Source: CAD feature listing. Evaluate the final solid. Frame: model axes, mm. Face numbers are marked on the shaded views. A direction names the side the tool comes from. Coordinates: 2 decimals unless noted, no trailing zeros. Order: outer loops, then holes, each group sorted by start corner. A loop starts at its lowest first (then second) coordinate and runs counter-clockwise, first axis right, second up. Notation, with made-up numbers: (-4.5, 62) - (54.5, 62) arc R11 ccw to (54.5, 78) - close; hole circle Ø9 at (34.25, 73). An arc over 180 degrees is marked (long way). One line per question, with ' | ' between items. Start each with the question number.
(1) Section D-D (y = -7). Return the cut outline in (x, z) (1 decimal).
(2) Section C-C (z = -6.5). Return the cut outline in (x, y) (1 decimal), then the cut area to 3 significant figures.
(3) Section A-A (x = 11.5). Return the cut outline in (y, z), then the cut area to 3 significant figures.
(4) Line query: line 1 along X through (y, z) = (0, 3); line 2 along X through (y, z) = (0, 5.25); line 3 along Z through (x, y) = (10, 0). Output: solid intervals per line, ascending.
(5) Draft query along Y for the marked faces 1, 2, 3 and 4. Return one class per face: +Y half, -Y half, draft (parallel to the pull), parting line (faces both ways), or undercut.
(6) Contact query for flat-ended pins moving along their axis: P1, Ø6.5, axis at y = 0, z = 0, coming from the +X side; P2, Ø6, axis at x = 11.5, z = 7, coming from the +Y side; P3, Ø1.5, axis at x = 27, z = -1, coming from the +Y side; P4, Ø4, axis at x = 19, y = -1.5, coming from the +Z side. Output: stop coordinate, or through.
(7) Section B-B (y = 0). Count the separate pieces of the cut face and the enclosed holes in it, then the cut area to 3 significant figures.
(8) Access query for the marked faces 5, 6 and 7. Directions: +Z, -Z, +X, -X, +Y, -Y. A direction counts if a zero-diameter tool reaches every point of the face in a straight line with its end or side. Return the directions, or none.
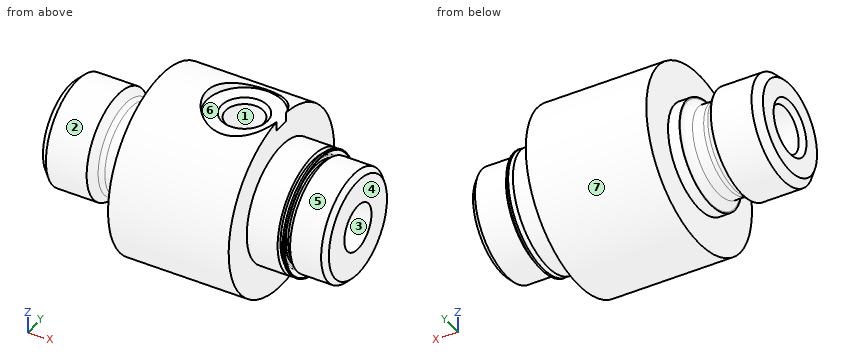
Autodesk Inventor part; units mm, degrees
ref_plane "dp1_XY" through (9.525, 5.5245, 0) normal (0, 0, 1) x (1, 0, 0)
ref_plane "dp1_YZ" through (9.525, 5.5245, 0) normal (1, 0, 0) x (0, 1, 0)
ref_plane "dp1_ZX" through (9.525, 5.5245, 0) normal (0, 1, 0) x (0, 0, 1)
sketch "Sketch_2" plane through (0, 0, 0) normal (0, 0, 1) x (1, 0, 0)
  line L0 (9.525, 0) -> (0, 0)
  line L1 (0, 0) -> (0, 4.8006)
  line L2 (0, 4.8006) -> (0.7557, 5.5563)
  line L3 (0.7557, 5.5563) -> (5.0286, 5.5563)
  line L4 (5.0286, 5.5563) -> (5.7864, 4.8042)
  arc A0 (5.7864, 4.8042) -> (6.35, 4.572) centre (6.35, 5.3721) ccw
  line L5 (6.35, 4.572) -> (7.5184, 4.572)
  arc A1 (7.5184, 4.572) -> (8.3185, 5.3721) centre (7.5184, 5.3721) ccw
  line L6 (8.3185, 5.3721) -> (8.3185, 5.5245)
  line L7 (8.3185, 5.5245) -> (9.525, 5.5245)
  line L8 (9.525, 5.5245) -> (9.525, 0)
  line L9 (9.525, 0) -> (0, 0)
revolve "Revolution1" add sketch "Sketch_2" angle 360 about axis through (9.525, 0, 0) along (1, 0, 0)
thread "Thread1"
sketch "Sketch_3" plane through (0, 0, 0) normal (0, 0, 1) x (1, 0, 0)
  line L0 (30.1752, 0) -> (9.525, 0)
  line L1 (9.525, 0) -> (9.525, 9.3726)
  line L2 (9.525, 9.3726) -> (25.4, 9.3726)
  line L3 (25.4, 9.3726) -> (25.4, 5.1626)
  line L4 (25.4, 5.1626) -> (25.908, 5.1626)
  line L5 (25.908, 5.1626) -> (26.416, 5.6706)
  line L6 (26.416, 5.6706) -> (29.6672, 5.6706)
  line L7 (29.6672, 5.6706) -> (30.1752, 5.1626)
  line L8 (30.1752, 5.1626) -> (30.1752, 0)
  line L9 (30.1752, 0) -> (9.525, 0)
revolve "Revolution2" add sketch "Sketch_3" angle 360 about axis through (30.1752, 0, 0) along (1, 0, 0)
sketch "Sketch3" plane through (0, 0, 0) normal (-1, 0, 0) x (0, 0, 1)
  point P0 (0, 0)
hole "Hole1" at (0, 0, 0) direction (1, 0, 0) diameter 4.8133 depth 30.1752 countersink diameter 5.8293 countersink angle 90
sketch "Sketch_12" plane through (0, 0, 0) normal (0, 1, 0) x (-1, 0, 0)
  line L0 (-18.288, 9.3726) -> (-18.288, -1.016)
  line L1 (-18.288, -1.016) -> (-20.2717, -1.016)
  line L2 (-20.2717, -1.016) -> (-20.2717, 7.9273)
  line L3 (-20.2717, 7.9273) -> (-20.701, 8.3566)
  line L4 (-20.701, 8.3566) -> (-22.2504, 8.3566)
  line L5 (-22.2504, 8.3566) -> (-22.2504, 9.3726)
  line L6 (-22.2504, 9.3726) -> (-18.288, 9.3726)
  line L7 (-18.288, 9.3726) -> (-18.288, -1.016)
revolve "Revolution3" cut sketch "Sketch_12" angle 360 about axis through (18.288, 0, 9.3726) along (0, 0, 1)
thread "Thread2"
sketch "Sketch_14" plane through (0, 0, 0) normal (0, 0, 1) x (1, 0, 0)
  line L0 (25.4, 0) -> (22.1615, 0)
  line L1 (22.1615, 6.1659) -> (25.4, 6.1659)
  line L2 (25.4, 6.1659) -> (25.4, 9.9758)
  line L3 (25.4, 9.9758) -> (22.1615, 9.9758)
  line L4 (22.1615, 9.9758) -> (22.1615, 6.1659)
revolve "Revolution4" cut sketch "Sketch_14" angle 360 about axis through (25.4, 0, 0) along (1, 0, 0)
sketch "Sketch_47" plane through (0, 0, 0) normal (0, 0, 1) x (1, 0, 0)
  line L0 (25.908, 0) -> (25.4, 0)
  line L1 (25.4, 4.9085) -> (25.908, 4.9085)
  line L2 (25.908, 4.9085) -> (25.908, 5.1626)
  line L3 (25.908, 5.1626) -> (25.654, 5.1626)
  line L4 (25.654, 5.1626) -> (25.5116, 5.305)
  arc A0 (25.5116, 5.4846) -> (25.5116, 5.305) centre (25.6014, 5.3948) ccw
  line L5 (25.5116, 5.4846) -> (26.1087, 6.0817)
  line L6 (26.1087, 6.0817) -> (26.1087, 6.1659)
  line L7 (26.1087, 6.1659) -> (25.9055, 6.1659)
  line L8 (25.9055, 6.1659) -> (25.4, 5.6603)
  line L9 (25.4, 5.6603) -> (25.4, 4.9085)
revolve "Revolution5" add sketch "Sketch_47" angle 360 about axis through (25.908, 0, 0) along (1, 0, 0)
ref_plane "dp1_XY" through (9.525, 5.5245, 0) normal (0, 0, 1) x (1, 0, 0)
ref_plane "dp1_YZ" through (9.525, 5.5245, 0) normal (1, 0, 0) x (0, 1, 0)
ref_plane "dp1_ZX" through (9.525, 5.5245, 0) normal (0, 1, 0) x (0, 0, 1)
ref_plane "dp2_XY" through (9.525, -5.5245, 0) normal (0, 0, 1) x (1, 0, 0)
ref_plane "dp2_YZ" through (9.525, -5.5245, 0) normal (1, 0, 0) x (0, 1, 0)
ref_plane "dp2_ZX" through (9.525, -5.5245, 0) normal (0, 1, 0) x (0, 0, 1)
ref_plane "port_XY" through (18.288, 0, 0) normal (0, 0, 1) x (1, 0, 0)
ref_plane "port_YZ" through (18.288, 0, 0) normal (1, 0, 0) x (0, 1, 0)
ref_plane "port_ZX" through (18.288, 0, 0) normal (0, 1, 0) x (0, 0, 1)
ref_plane "rod_guide_XY" through (0, 0, 0) normal (1, 0, 0) x (0, 0, -1)
ref_plane "rod_guide_YZ" through (0, 0, 0) normal (0, 0, -1) x (0, 1, 0)
ref_plane "rod_guide_ZX" through (0, 0, 0) normal (0, 1, 0) x (1, 0, 0)
ref_plane "s1_XY" through (8.3185, 0, 0) normal (0, 0, 1) x (1, 0, 0)
ref_plane "s1_YZ" through (8.3185, 0, 0) normal (1, 0, 0) x (0, 1, 0)
ref_plane "s1_ZX" through (8.3185, 0, 0) normal (0, 1, 0) x (0, 0, 1)
ref_plane "s2_XY" through (9.525, 0, 0) normal (0, 0, 1) x (1, 0, 0)
ref_plane "s2_YZ" through (9.525, 0, 0) normal (1, 0, 0) x (0, 1, 0)
ref_plane "s2_ZX" through (9.525, 0, 0) normal (0, 1, 0) x (0, 0, 1)
ref_plane "t1_XY" through (9.525, 0, 0) normal (1, 0, 0) x (0, 0, -1)
ref_plane "t1_YZ" through (9.525, 0, 0) normal (0, 0, -1) x (0, 1, 0)
ref_plane "t1_ZX" through (9.525, 0, 0) normal (0, 1, 0) x (1, 0, 0)
ref_plane "t111_XY" through (9.525, 0, 0) normal (1, 0, 0) x (0, 0, -1)
ref_plane "t111_YZ" through (9.525, 0, 0) normal (0, 0, -1) x (0, 1, 0)
ref_plane "t111_ZX" through (9.525, 0, 0) normal (0, 1, 0) x (1, 0, 0)
ref_plane "to_foot_bracket_XY" through (9.525, 0, 0) normal (1, 0, 0) x (0, 0, -1)
ref_plane "to_foot_bracket_YZ" through (9.525, 0, 0) normal (0, 0, -1) x (0, 1, 0)
ref_plane "to_foot_bracket_ZX" through (9.525, 0, 0) normal (0, 1, 0) x (1, 0, 0)
ref_plane "to_nut_XY" through (8.3185, 0, 0) normal (1, 0, 0) x (0, 0, -1)
ref_plane "to_nut_YZ" through (8.3185, 0, 0) normal (0, 0, -1) x (0, 1, 0)
ref_plane "to_nut_ZX" through (8.3185, 0, 0) normal (0, 1, 0) x (1, 0, 0)
ref_plane "to_rod_XY" through (0, 0, 0) normal (1, 0, 0) x (0, 0, -1)
ref_plane "to_rod_YZ" through (0, 0, 0) normal (0, 0, -1) x (0, 1, 0)
ref_plane "to_rod_ZX" through (0, 0, 0) normal (0, 1, 0) x (1, 0, 0)
ref_plane "to_screw_XY" through (18.288, 0, 0) normal (0, 1, 0) x (1, 0, 0)
ref_plane "to_screw_YZ" through (18.288, 0, 0) normal (1, 0, 0) x (0, 0, -1)
ref_plane "to_screw_ZX" through (18.288, 0, 0) normal (0, 0, -1) x (0, 1, 0)
ref_plane "to_trunnion_brackets_XY" through (7.9248, 0, 0) normal (0, 1, 0) x (1, 0, 0)
ref_plane "to_trunnion_brackets_YZ" through (7.9248, 0, 0) normal (1, 0, 0) x (0, 0, -1)
ref_plane "to_trunnion_brackets_ZX" through (7.9248, 0, 0) normal (0, 0, -1) x (0, 1, 0)
ref_plane "to_trunnion_brackets1_XY" through (7.9248, 9.525, 0) normal (0, 1, 0) x (1, 0, 0)
ref_plane "to_trunnion_brackets1_YZ" through (7.9248, 9.525, 0) normal (1, 0, 0) x (0, 0, -1)
ref_plane "to_trunnion_brackets1_ZX" through (7.9248, 9.525, 0) normal (0, 0, -1) x (0, 1, 0)
ref_plane "to_trunnion_brackets2_XY" through (7.9248, -9.525, 0) normal (0, 1, 0) x (1, 0, 0)
ref_plane "to_trunnion_brackets2_YZ" through (7.9248, -9.525, 0) normal (1, 0, 0) x (0, 0, -1)
ref_plane "to_trunnion_brackets2_ZX" through (7.9248, -9.525, 0) normal (0, 0, -1) x (0, 1, 0)
ref_plane "to_tube_XY" through (25.908, 0, 0) normal (1, 0, 0) x (0, 0, -1)
ref_plane "to_tube_YZ" through (25.908, 0, 0) normal (0, 0, -1) x (0, 1, 0)
ref_plane "to_tube_ZX" through (25.908, 0, 0) normal (0, 1, 0) x (1, 0, 0)
properties part number "01R000-0_rod_guide"
Response values:
1) outline: (9.5, -6.2) - (22.2, -6.2) - (22.2, 6.2) - (9.5, 6.2) - close
2) outline: (9.5, -6.8) - (22.2, -6.8) - (22.2, 6.8) - (9.5, 6.8) - close | area: 171 mm²
3) outline: circle Ø18.75 at (0, 0); hole circle Ø4.81 at (0, 0) | area: 258 mm²
4) line 1: x = 0 to 16.3, 20.27 to 30.18 | line 2: x = 0.45 to 5.34, 8.31 to 16.3, 20.27 to 25.57, 26 to 30.09 | line 3: z = -9.37 to -2.41, 2.41 to 9.37
5) face 1: undercut | face 2: parting line | face 3: undercut | face 4: draft
6) P1: stops at x = 30.18 | P2: stops at y = 8.48 | P3: stops at y = 5.67 | P4: stops at z = 8.36
7) separate pieces: 3 | enclosed holes: 0 | area: 253 mm²
8) face 5: +X | face 6: +Z | face 7: +X, -X
